The figure shows three views and two pictorial views of one solid part (mm, origin at its lowest corner). Answer the questions. A direction names the side the tool comes from. Give positions to 0.01 mm unless a question says otherwise; leave off trailing zeros. Loops run counter-clockwise (first coordinate to the right, second up) from the corner with the lowest first, then second, coordinate; pieces in that order, holes last. Notation, with made-up numbers: M -3,79 L 35,79 A22 cw 35,103 Z; hole C -16.5,51 d8. An arc over 180 degrees is marked long. Answer as a JSON object with one key per item and string values. Group by question number.
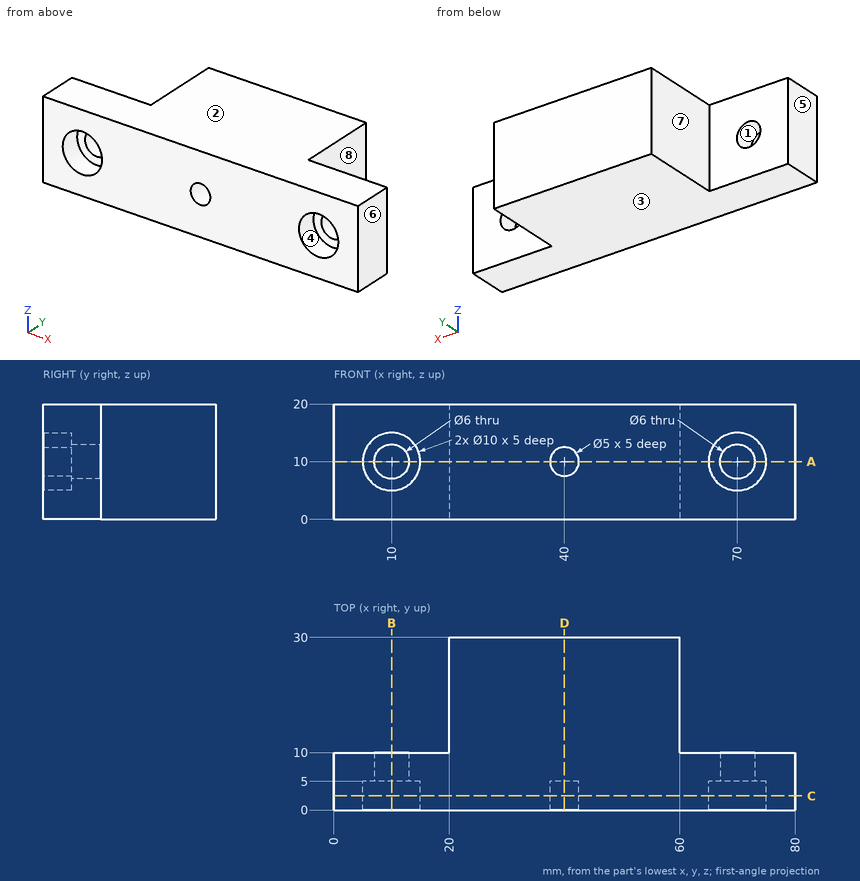
Item 1: A cutting plane is placed at B-B (x = 10). Determine the outline of the cut face in (y, z).
Item 2: A cutting plane is placed at A-A (z = 10). Determine the outline of the cut face in (x, y), and give its area (4 significant figures).
Item 3: A tool of negligible diameter and unlimited length cuts with its end or side. For the marked faces 4, 5, 6, 7 and 8, from which of +Z, -Z, +X, -X, +Y, -Y can it reach the whole face along a straight path? Write none if from no direction.
Item 4: Find the intervals of material crossed by probe 1 along X at (y, z) = (8.5, 10); probe 2 along X at (y, z) = (3.6, 10); probe 3 along Z at (x, y) = (11.5, 4), in increasing order. Write a range as [from, to].
Item 5: For a pull along Z with two mould halves and no side action, classify the marked faces 1, 2 and 3 as pulls with the +Z half, pulls with the -Z half, needs draft (parallel to the pull), parting line crosses it, or undercut.
Item 6: A cutting plane is placed at C-C (y = 2.5). Determine the outline of the cut face in (x, z).
Item 7: Given pin 1 Ø3 at (x, z) = (72, 10) entering from -Y; pin 2 Ø5.5 at (x, z) = (70, 10) entering from +Y; pin 3 Ø2 at (x, z) = (20.5, 9.5) entering from -Y; pin 4 Ø2 at (y, z) = (17.5, 5.5) entering from +X, each flat-ended and moving along its own axis, determine where each tip first touches the part or whether it passes through.
Item 8: A cutting plane is placed at D-D (x = 40). Determine the outline of the cut face in (y, z), and give its area (3 significant figures).
The answers:
{
 "1": {"outline": "M 0,0 L 10,0 L 10,7 L 5,7 L 5,5 L 0,5 Z; M 0,15 L 5,15 L 5,13 L 10,13 L 10,20 L 0,20 Z"},
 "2": {"outline": "M 0,0 L 5,0 L 5,5 L 7,5 L 7,10 L 0,10 Z; M 13,5 L 15,5 L 15,0 L 37.5,0 L 37.5,5 L 42.5,5 L 42.5,0 L 65,0 L 65,5 L 67,5 L 67,10 L 60,10 L 60,30 L 20,30 L 20,10 L 13,10 Z; M 73,5 L 75,5 L 75,0 L 80,0 L 80,10 L 73,10 Z", "area": "1,415 mm^2"},
 "3": {"face 4": "-Y", "face 5": "+Z, -Z, -X, +Y, -Y", "face 6": "+Z, -Z, +X, +Y, -Y", "face 7": "+Z, -Z, -X, +Y", "face 8": "+Z, -Z, +X, +Y"},
 "4": {"probe 1": "x = [0, 7], [13, 67], [73, 80]", "probe 2": "x = [0, 5], [15, 37.5], [42.5, 65], [75, 80]", "probe 3": "z = [0, 5.23], [14.77, 20]"},
 "5": {"face 1": "undercut", "face 2": "pulls with the +Z half", "face 3": "pulls with the -Z half"},
 "6": {"outline": "M 0,0 L 80,0 L 80,20 L 0,20 Z; hole C 10,10 d10; hole C 40,10 d5; hole C 70,10 d10"},
 "7": {"pin 1": "stops at y = 5", "pin 2": "passes through", "pin 3": "stops at y = 0", "pin 4": "stops at x = 60"},
 "8": {"outline": "M 0,0 L 30,0 L 30,20 L 0,20 L 0,12.5 L 5,12.5 L 5,7.5 L 0,7.5 Z", "area": "575 mm^2"}
}
